Read the model definition and answer for the solid it produces. Units are mm, in the model's axes. Face numbers are marked on the shaded views. Give positions to 0.01 mm unless a question says otherwise; leave off trailing zeros. Order: outer loops, then holes, each group sorted by start corner. A loop starts at its lowest first (then second) coordinate and runs counter-clockwise, first axis right, second up. Notation, with made-up numbers: (4.5, 76.5) -> (41.5, 76.5) arc R14 ccw to (41.5, 91.5) -> close; hole circle Ø4 at (28.25, 88.5). An arc over 180 degrees is marked (long way). Answer as CSV lines item,"result". Start each with the question number.
1) Find section C-C (x = 11.5). Determine the outline of the cut face in (y, z).
2) Find section A-A (x = 0). Determine the outline of the cut face in (y, z).
3) The mould has two halves that part along X. Classify the marked faces 1, 2 and 3: +X half, -X half, draft (parallel to the pull), parting line (faces both ways), or undercut.
4) Straight lines are drawn through the part: L1, parallel to Y at x = 0, z = 1.45; L2, parallel to X at y = 12.5, z = 0.4; L3, parallel to X at y = 0.5, z = 2.75. For each, find the intervals that lie inside material, in ascending order. Write a range as from..to.
5) Find section D-D (z = 2.95). Determine the outline of the cut face in (x, y), and give its area (3 significant figures).
6) Find section B-B (x = 22.5). Determine the outline of the cut face in (y, z).
7) Flat-ended cylindrical pins translate along their axes: pin 1 Ø1.5 at (x, z) = (-21.5, 3) entering from +Y; pin 2 Ø1 at (y, z) = (-16.5, 1.5) entering from -X; pin 3 Ø9 at (x, y) = (-20.63, 11.91) entering from +Z. Find the tip coordinate at first contact, or state that the pin passes through.
```python
from build123d import *

# Parameters (mm, degrees)
SKETCH1_R           = 28.9052
SKETCH1_R_2         = 2.8067
SKETCH1_R_3         = 18.7452
BOSS_EXTRUDE1_DEPTH = 4.318


with BuildPart() as part:
    # Sketch1 → Boss-Extrude1 (new body)
    with BuildSketch(Plane.XY):
        Circle(SKETCH1_R)
        with Locations((0, 23.8252)):
            Circle(SKETCH1_R_2, mode=Mode.SUBTRACT)
        with Locations((20.63322845, 11.9126)):
            Circle(SKETCH1_R_2, mode=Mode.SUBTRACT)
        with Locations((20.63322845, -11.9126)):
            Circle(SKETCH1_R_2, mode=Mode.SUBTRACT)
        with Locations((0, -23.8252)):
            Circle(SKETCH1_R_2, mode=Mode.SUBTRACT)
        with Locations((-20.63322845, -11.9126)):
            Circle(SKETCH1_R_2, mode=Mode.SUBTRACT)
        with Locations((-20.63322845, 11.9126)):
            Circle(SKETCH1_R_2, mode=Mode.SUBTRACT)
        Circle(SKETCH1_R_3, mode=Mode.SUBTRACT)
    extrude(amount=BOSS_EXTRUDE1_DEPTH)


solid = part.part
```
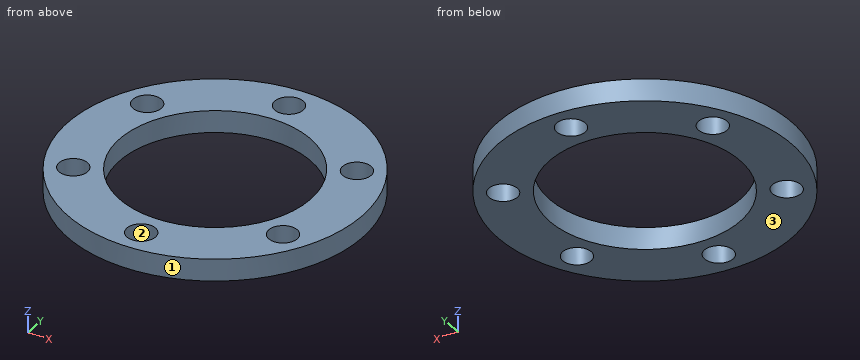
Findings below:
1,outline,"(-26.52, 0) -> (-14.8, 0) -> (-14.8, 4.32) -> (-26.52, 4.32) -> close; (14.8, 0) -> (26.52, 0) -> (26.52, 4.32) -> (14.8, 4.32) -> close"
2,outline,"(-28.91, 0) -> (-26.63, 0) -> (-26.63, 4.32) -> (-28.91, 4.32) -> close; (-21.02, 0) -> (-18.75, 0) -> (-18.75, 4.32) -> (-21.02, 4.32) -> close; (18.75, 0) -> (21.02, 0) -> (21.02, 4.32) -> (18.75, 4.32) -> close; (26.63, 0) -> (28.91, 0) -> (28.91, 4.32) -> (26.63, 4.32) -> close"
3,face 1,"parting line"
3,face 2,"undercut"
3,face 3,"draft"
4,L1,"-28.91..-26.63, -21.02..-18.75, 18.75..21.02, 26.63..28.91"
4,L2,"-26.06..-23.38, -17.89..-13.97, 13.97..17.89, 23.38..26.06"
4,L3,"-28.9..-18.74, 18.74..28.9"
5,outline,"circle Ø57.81 at (0, 0); hole circle Ø5.61 at (-20.63, -11.91); hole circle Ø5.61 at (-20.63, 11.91); hole circle Ø37.49 at (0, 0); hole circle Ø5.61 at (0, -23.83); hole circle Ø5.61 at (0, 23.83); hole circle Ø5.61 at (20.63, -11.91); hole circle Ø5.61 at (20.63, 11.91)"
5,area,"1,370 mm²"
6,outline,"(-18.15, 0) -> (-14.01, 0) -> (-14.01, 4.32) -> (-18.15, 4.32) -> close; (-9.82, 0) -> (9.82, 0) -> (9.82, 4.32) -> (-9.82, 4.32) -> close; (14.01, 0) -> (18.15, 0) -> (18.15, 4.32) -> (14.01, 4.32) -> close"
7,pin 1,"y = 20.12"
7,pin 2,"x = -24.07"
7,pin 3,"z = 4.32"
